Part model, mm, in its own coordinate system. A direction names the side the tool comes from. Give positions to 0.01 mm unless a question says otherwise; leave off trailing zeros. Write each loop counter-clockwise with the first axis right and the second up, starting at its lowest first coordinate (ties: lowest second). Pieces come first, ordered by that corner, then holes.
```python
from build123d import *

# Parameters (mm, degrees)
F0_W      = 171.45
F0_H      = 158.75
F0_W_2    = 165.1
F0_H_2    = 152.4
F1_DEPTH  = 609.6
F3_DEPTH  = 158.751
F4_W      = 203.2
F4_H      = 284.28666
F4_R      = 3.175
F4_W_2    = 152.4
F4_H_2    = 233.48666
F4_H_3    = 25.4
F5_DEPTH  = 4.7625
F6_W      = 152.4
F6_H      = 101.6
F7_DEPTH  = 25.4
F8_W      = 160.3375
F8_H      = 4.7625
F9_DEPTH  = 4.7625
F10_W     = 160.3375
F10_H     = 4.7625
F11_DEPTH = 4.7625


with BuildPart() as f1:
    # F0 (on Top) → F1 (new body)
    with BuildSketch(Plane.XY):
        Rectangle(F0_W, F0_H)
        Rectangle(F0_W_2, F0_H_2, mode=Mode.SUBTRACT)
    extrude(amount=F1_DEPTH)

    # F2 (on face) → F3 (cut, through all)
    with BuildSketch(Plane.XZ.offset(79.375)):
        Polygon((-85.725, 438.15), (85.725, 609.6), (-85.725, 609.6), align=None)
    extrude(amount=-F3_DEPTH, mode=Mode.SUBTRACT)

    # F4 (on face) → F5 (join)
    with BuildSketch(Plane(origin=(-261.9375, 0, 261.9375), x_dir=(0, -1, 0), z_dir=(-0.707107, 0, 0.707107))):
        with Locations((0, 370.435565)):
            Rectangle(F4_W, F4_H)
        with Locations((-88.9, 240.992235)):
            Circle(F4_R, mode=Mode.SUBTRACT)
        with Locations((0, 240.992235)):
            Circle(F4_R, mode=Mode.SUBTRACT)
        with Locations((88.9, 240.992235)):
            Circle(F4_R, mode=Mode.SUBTRACT)
        with Locations((-88.9, 370.435565)):
            Circle(F4_R, mode=Mode.SUBTRACT)
        with Locations((0, 370.435565)):
            Rectangle(F4_W_2, F4_H_2, mode=Mode.SUBTRACT)
        with Locations((-88.9, 499.878895)):
            Circle(F4_R, mode=Mode.SUBTRACT)
        with Locations((0, 499.878895)):
            Circle(F4_R, mode=Mode.SUBTRACT)
        with Locations((88.9, 368.56214)):
            Circle(F4_R, mode=Mode.SUBTRACT)
        with Locations((88.9, 499.878895)):
            Circle(F4_R, mode=Mode.SUBTRACT)
        with Locations((0, 215.592235)):
            Rectangle(F4_W, F4_H_3)
        with Locations((-50.8, 215.592235)):
            Circle(F4_R, mode=Mode.SUBTRACT)
        with Locations((50.8, 215.592235)):
            Circle(F4_R, mode=Mode.SUBTRACT)
    extrude(amount=F5_DEPTH)

    # F6 (on face) → F7 (cut)
    with BuildSketch(Plane.YZ.offset(85.725)):
        with Locations((0, 365.125)):
            Rectangle(F6_W, F6_H)
    extrude(amount=-F7_DEPTH, mode=Mode.SUBTRACT)

    # F8 (on face) → F9 (join)
    with BuildSketch(Plane(origin=(0, -76.2, 0), x_dir=(-1, 0, 0), z_dir=(0, 1, 0))):
        with Locations((2.38125, 311.94375)):
            Rectangle(F8_W, F8_H)
    extrude(amount=F9_DEPTH)

    # F10 (on face) → F11 (join)
    with BuildSketch(Plane.XZ.offset(-76.2)):
        with Locations((-2.38125, 311.94375)):
            Rectangle(F10_W, F10_H)
    extrude(amount=F11_DEPTH)


solid = f1.part
```
1) 3-axis set-ups, long thin cutter, end or side, ignore diameter. For faces 4 (the face through (82.55, -1, 155)), 5 (the face through (5, 76.2, 293)), 6 (the face through (-1, 79.375, 233)): which of +Z, -Z, +X, -X, +Y, -Y reach the whole face in a straight line?
Answers follow:
face 4: -Z
face 5: none
face 6: -Z, +X, +Y
2) Wall check: L1, parallel to Y at x = 3, z = 343 (3 decimals); L2, parallel to X at y = -17, z = 95 (3 decimals); L3, parallel to X at y = -32, z = 567.5 (3 decimals). Give the ranges that are in metal, low to high.
Answers follow:
L1: y = -79.375 to -76.2, 76.2 to 79.375
L2: x = -85.725 to -82.55, 82.55 to 85.725
L3: x = 82.55 to 85.725
3) Saw through at C-C, the plane z = 376.5. Write the cut outline in (x, y) (3 decimals), then the cut area to 3 significant figures.
Answers follow:
outline: (-85.725, -79.375) - (85.725, -79.375) - (85.725, -76.2) - (-82.55, -76.2) - (-82.55, 76.2) - (85.725, 76.2) - (85.725, 79.375) - (-85.725, 79.375) - close
area: 1,570 mm2
4) Two-plate mould, pull along Y, no slides. Class faces 1 (the face through (85.725, -1, 301)), 2 (the face through (5, -76.2, 293)), 3 (the face through (-1, -79.375, 233)): +Y half, -Y half, draft (parallel to the pull), parting line (faces both ways), or undercut.
Answers follow:
face 1: draft
face 2: undercut
face 3: -Y half
5) Saw through at A-A, the plane x = 41. Write the cut outline in (y, z) (1 decimal), then the cut area to 3 significant figures.
Answers follow:
outline: (-101.6, 564.9) - (-79.4, 564.9) - (-79.4, 0) - (-76.2, 0) - (-76.2, 309.6) - (-71.4, 309.6) - (-71.4, 314.3) - (-76.2, 314.3) - (-76.2, 571.6) - (-101.6, 571.6) - close; (71.4, 309.6) - (76.2, 309.6) - (76.2, 0) - (79.4, 0) - (79.4, 564.9) - (101.6, 564.9) - (101.6, 571.6) - (76.2, 571.6) - (76.2, 314.3) - (71.4, 314.3) - close
area: 3,970 mm2
6) Pin check, flat tips, straight feed: pin 1 Ø2.5 at (y, z) = (-73.5, 312) entering from +X (3 decimals); pin 2 Ø12 at (x, y) = (-99.5, -26) entering from -Z (3 decimals); pin 3 Ø1 at (x, y) = (84, 2.5) entering from +Z. Stop position of each tip, or through.
Answers follow:
pin 1: stops at x = 85.725
pin 2: stops at z = 418.375
pin 3: stops at z = 615.11
7) Saw through at B-B, the plane y = 13. Write the cut outline in (x, z) (3 decimals), then the cut area to 3 significant figures.
Answers follow:
outline: (-121.839, 408.772) - (-118.471, 405.404) - (-85.725, 438.15) - (-85.725, 0) - (-82.55, 0) - (-82.55, 441.325) - (-85.918, 444.693) - close; (79.182, 609.793) - (82.55, 606.425) - (82.55, 415.925) - (85.725, 415.925) - (85.725, 609.6) - (100.511, 624.386) - (97.143, 627.753) - close; (82.55, 0) - (85.725, 0) - (85.725, 314.325) - (82.55, 314.325) - close
area: 3,370 mm2
8) Saw through at D-D, the plane z = 93.5. Write the cut outline in (x, y) (3 decimals), then the cut area to 3 significant figures.
Answers follow:
outline: (-85.725, -79.375) - (85.725, -79.375) - (85.725, 79.375) - (-85.725, 79.375) - close; hole (-82.55, -76.2) - (82.55, -76.2) - (82.55, 76.2) - (-82.55, 76.2) - close
area: 2,060 mm2
